from build123d import *

# Parameters (mm, degrees)
EXTRUDE_1_DEPTH     = 15
SKETCH_3_W          = 10.742953118
SKETCH_3_H          = 10
EXTRUDE_2_DEPTH     = 57.5
SKETCH_4_W          = 10.742953118
SKETCH_4_H          = 5
EXTRUDE_3_DEPTH     = 57.5
CUT_EXTRUDE_1_REACH = 133.077
SKETCH_5_R          = 1.65
CUT_EXTRUDE_2_REACH = 137.116
SKETCH_6_R          = 1.7
CUT_EXTRUDE_3_REACH = 135.143
SKETCH_7_R          = 1.5
CHAMFER_1_SIZE      = 5
CHAMFER_2_SIZE      = 2
CHAMFER_3_SIZE      = 5
CHAMFER_4_SIZE      = 1


with BuildPart() as part:
    # Sketch 1 → Extrude 1 (new body)
    with BuildSketch(Plane.XY):
        Polygon((0, 110), (0, 0), (-30, 0), (-30, 5), (-20, 5), (-10.742953118, 14.257046882), (-10.742953118, 110), align=None)
    extrude(amount=EXTRUDE_1_DEPTH)


with BuildPart() as body_2:
    # Mirror 9: mirrored copy
    add(part.part.mirror(Plane.XY.offset(-28.75)))


with BuildPart() as part_1:
    add(part.part)

    add(body_2.part)  # Extrude 2 merges body 2
    # Sketch 3 → Extrude 2 (add)
    with BuildSketch(Plane.XY.offset(-57.5)):
        with Locations((-5.371476559, 75)):
            Rectangle(SKETCH_3_W, SKETCH_3_H)
    extrude(amount=EXTRUDE_2_DEPTH)

    # Sketch 4 → Extrude 3 (add)
    with BuildSketch(Plane.XY.offset(-57.5)):
        with Locations((-5.371476559, 2.5)):
            Rectangle(SKETCH_4_W, SKETCH_4_H)
    extrude(amount=EXTRUDE_3_DEPTH)

    # Sketch 5 → Cut-Extrude 1 (cut, up to next)
    with BuildSketch(Plane(origin=(0, 5, 0), x_dir=(1, 0, 0), z_dir=(0, 1, 0)), mode=Mode.PRIVATE) as cut_extrude_1_sk1:
        with Locations(Location((-24.537178605, 65, 0), (0, 0, 270))):
            Circle(SKETCH_5_R)
    cut_extrude_1_tool1 = extrude(cut_extrude_1_sk1.sketch, amount=-CUT_EXTRUDE_1_REACH, mode=Mode.PRIVATE) & part_1.part
    # Sketch 5 → Cut-Extrude 1 (cut, up to next)
    with BuildSketch(Plane(origin=(0, 5, 0), x_dir=(1, 0, 0), z_dir=(0, 1, 0)), mode=Mode.PRIVATE) as cut_extrude_1_sk2:
        with Locations(Location((-24.537178605, -7.5, 0), (0, 0, 270))):
            Circle(SKETCH_5_R)
    cut_extrude_1_tool2 = extrude(cut_extrude_1_sk2.sketch, amount=-CUT_EXTRUDE_1_REACH, mode=Mode.PRIVATE) & part_1.part
    add(cut_extrude_1_tool1.solids().sort_by_distance((-24.537179, 5, -65))[0], mode=Mode.SUBTRACT)
    add(cut_extrude_1_tool2.solids().sort_by_distance((-24.537179, 5, 7.5))[0], mode=Mode.SUBTRACT)

    # Sketch 6 → Cut-Extrude 2 (cut, up to next)
    with BuildSketch(Plane.XZ, mode=Mode.PRIVATE) as cut_extrude_2_sk1:
        with Locations((-4.537178605, -7.5)):
            Circle(SKETCH_6_R)
    cut_extrude_2_tool1 = extrude(cut_extrude_2_sk1.sketch, amount=-CUT_EXTRUDE_2_REACH, mode=Mode.PRIVATE) & part_1.part
    # Sketch 6 → Cut-Extrude 2 (cut, up to next)
    with BuildSketch(Plane.XZ, mode=Mode.PRIVATE) as cut_extrude_2_sk2:
        with Locations((-4.537178605, -50)):
            Circle(SKETCH_6_R)
    cut_extrude_2_tool2 = extrude(cut_extrude_2_sk2.sketch, amount=-CUT_EXTRUDE_2_REACH, mode=Mode.PRIVATE) & part_1.part
    add(cut_extrude_2_tool1.solids().sort_by_distance((-4.537179, 0, -7.5))[0], mode=Mode.SUBTRACT)
    add(cut_extrude_2_tool2.solids().sort_by_distance((-4.537179, 0, -50))[0], mode=Mode.SUBTRACT)

    # Sketch 7 → Cut-Extrude 3 (cut, up to next)
    with BuildSketch(Plane.ZY.offset(10.742953118), mode=Mode.PRIVATE) as cut_extrude_3_sk1:
        with Locations((-66.25, 100.05)):
            Circle(SKETCH_7_R)
    cut_extrude_3_tool1 = extrude(cut_extrude_3_sk1.sketch, amount=-CUT_EXTRUDE_3_REACH, mode=Mode.PRIVATE) & part_1.part
    # Sketch 7 → Cut-Extrude 3 (cut, up to next)
    with BuildSketch(Plane.ZY.offset(10.742953118), mode=Mode.PRIVATE) as cut_extrude_3_sk2:
        with Locations((8.75, 100.05)):
            Circle(SKETCH_7_R)
    cut_extrude_3_tool2 = extrude(cut_extrude_3_sk2.sketch, amount=-CUT_EXTRUDE_3_REACH, mode=Mode.PRIVATE) & part_1.part
    # Sketch 7 → Cut-Extrude 3 (cut, up to next)
    with BuildSketch(Plane.ZY.offset(10.742953118), mode=Mode.PRIVATE) as cut_extrude_3_sk3:
        with Locations((-66.25, 78.05)):
            Circle(SKETCH_7_R)
    cut_extrude_3_tool3 = extrude(cut_extrude_3_sk3.sketch, amount=-CUT_EXTRUDE_3_REACH, mode=Mode.PRIVATE) & part_1.part
    # Sketch 7 → Cut-Extrude 3 (cut, up to next)
    with BuildSketch(Plane.ZY.offset(10.742953118), mode=Mode.PRIVATE) as cut_extrude_3_sk4:
        with Locations(Location((8.75, 78.05, 0), (0, 0, 270))):
            Circle(SKETCH_7_R)
    cut_extrude_3_tool4 = extrude(cut_extrude_3_sk4.sketch, amount=-CUT_EXTRUDE_3_REACH, mode=Mode.PRIVATE) & part_1.part
    add(cut_extrude_3_tool1.solids().sort_by_distance((-10.742953, 100.05, -66.25))[0], mode=Mode.SUBTRACT)
    add(cut_extrude_3_tool2.solids().sort_by_distance((-10.742953, 100.05, 8.75))[0], mode=Mode.SUBTRACT)
    add(cut_extrude_3_tool3.solids().sort_by_distance((-10.742953, 78.05, -66.25))[0], mode=Mode.SUBTRACT)
    add(cut_extrude_3_tool4.solids().sort_by_distance((-10.742953, 78.05, 8.75))[0], mode=Mode.SUBTRACT)

    # Chamfer 1
    chamfer_1_edges = [part_1.edges().sort_by_distance(p)[0] for p in [
        (-5.371476559, 80, 0),
        (-5.371476559, 80, -57.5),
        (-5.371476559, 70, 0),
        (-5.371476559, 70, -57.5),
        (-5.371476559, 5, 0),
        (-5.371476559, 5, -57.5),
    ]]
    chamfer(chamfer_1_edges, length=CHAMFER_1_SIZE)

    # Chamfer 2
    chamfer_2_edges = [part_1.edges().sort_by_distance(p)[0] for p in [
        (-5.371476559, 110, 0),
        (-30, 2.5, 15),
        (-5.371476559, 110, -57.5),
        (-30, 2.5, -57.5),
        (-5.371476559, 110, -72.5),
        (-30, 2.5, -72.5),
        (-5.371476559, 110, 15),
        (-30, 2.5, 0),
    ]]
    chamfer(chamfer_2_edges, length=CHAMFER_2_SIZE)

    # Chamfer 3
    # the kernel refuses this chamfer: 5 mm, written as the material it adds along each edge
    with BuildSketch(Plane(origin=(-10.742953118, 22.85841494, 0), x_dir=(-0.9996219169112968, 0, 0.027495876610586372), z_dir=(0, -1, 0))) as chamfer_3_piece_1_section:
        Polygon((CHAMFER_3_SIZE * 0.999621916911, CHAMFER_3_SIZE * 0.0274958766106), (-CHAMFER_3_SIZE * 0.0274958766106, CHAMFER_3_SIZE * 0.999621916911), (0, 0), align=None)
    chamfer_3_piece_1 = extrude(amount=22.85841494, mode=Mode.PRIVATE)
    chamfer_3_piece_1 = split(chamfer_3_piece_1, bisect_by=Plane(origin=(-12.636913345, 5, -1.178868923), z_dir=(0, 1, 0)), keep=Keep.TOP, mode=Mode.PRIVATE)
    chamfer_3_piece_1 = split(chamfer_3_piece_1, bisect_by=Plane(origin=(-12.636913345, 7.862667434, -2.137332566), z_dir=(0, -0.7071067811865476, 0.7071067811865476)), keep=Keep.TOP, mode=Mode.PRIVATE)
    chamfer_3_piece_1 = split(chamfer_3_piece_1, bisect_by=Plane(origin=(-15.366354777, 9.633645223, -1.178868923), z_dir=(0.7071067811865488, -0.7071067811865464, 0)), keep=Keep.TOP, mode=Mode.PRIVATE)
    add(chamfer_3_piece_1)
    with BuildSketch(Plane(origin=(-10.742953118, 22.85841494, 0), x_dir=(-0.9996219169112968, 0, 0.027495876610586372), z_dir=(0, -1, 0))) as chamfer_3_piece_2_section:
        Polygon((CHAMFER_3_SIZE * 0.999621916911, CHAMFER_3_SIZE * 0.0274958766106), (-CHAMFER_3_SIZE * 0.0274958766106, CHAMFER_3_SIZE * 0.999621916911), (0, 0), align=None)
    chamfer_3_piece_2 = extrude(amount=22.85841494, mode=Mode.PRIVATE)
    chamfer_3_piece_2 = split(chamfer_3_piece_2, bisect_by=Plane(origin=(-12.391958981, 5, -1.648896507), z_dir=(0, -1, 0)), keep=Keep.TOP, mode=Mode.PRIVATE)
    chamfer_3_piece_2 = split(chamfer_3_piece_2, bisect_by=Plane(origin=(-12.391958981, 5.425526159, -4.574473841), z_dir=(0, -0.7071067811865476, 0.7071067811865476)), keep=Keep.TOP, mode=Mode.PRIVATE)
    add(chamfer_3_piece_2)
    with BuildSketch(Plane(origin=(-10.742953118, 0, -57.5), x_dir=(-0.9996219169112968, 0, -0.027495876610586317), z_dir=(0, 1, 0))) as chamfer_3_piece_3_section:
        Polygon((CHAMFER_3_SIZE * 0.999621916911, CHAMFER_3_SIZE * 0.0274958766106), (-CHAMFER_3_SIZE * 0.0274958766106, CHAMFER_3_SIZE * 0.999621916911), (0, 0), align=None)
    chamfer_3_piece_3 = extrude(amount=22.85841494, mode=Mode.PRIVATE)
    chamfer_3_piece_3 = split(chamfer_3_piece_3, bisect_by=Plane(origin=(-12.391958981, 5.425526159, -52.925526159), z_dir=(0, -0.7071067811865476, -0.7071067811865476)), keep=Keep.TOP, mode=Mode.PRIVATE)
    chamfer_3_piece_3 = split(chamfer_3_piece_3, bisect_by=Plane(origin=(-12.391958981, 5, -55.851103493), z_dir=(0, -1, 0)), keep=Keep.TOP, mode=Mode.PRIVATE)
    add(chamfer_3_piece_3)
    with BuildSketch(Plane(origin=(-10.742953118, 0, -57.5), x_dir=(-0.9996219169112968, 0, -0.027495876610586317), z_dir=(0, 1, 0))) as chamfer_3_piece_4_section:
        Polygon((CHAMFER_3_SIZE * 0.999621916911, CHAMFER_3_SIZE * 0.0274958766106), (-CHAMFER_3_SIZE * 0.0274958766106, CHAMFER_3_SIZE * 0.999621916911), (0, 0), align=None)
    chamfer_3_piece_4 = extrude(amount=22.85841494, mode=Mode.PRIVATE)
    chamfer_3_piece_4 = split(chamfer_3_piece_4, bisect_by=Plane(origin=(-12.636913345, 7.862667434, -55.362667434), z_dir=(0, -0.7071067811865476, -0.7071067811865476)), keep=Keep.TOP, mode=Mode.PRIVATE)
    chamfer_3_piece_4 = split(chamfer_3_piece_4, bisect_by=Plane(origin=(-15.366354777, 9.633645223, -56.321131077), z_dir=(0.7071067811865488, -0.7071067811865464, 0)), keep=Keep.TOP, mode=Mode.PRIVATE)
    chamfer_3_piece_4 = split(chamfer_3_piece_4, bisect_by=Plane(origin=(-12.636913345, 5, -56.321131077), z_dir=(0, 1, 0)), keep=Keep.TOP, mode=Mode.PRIVATE)
    add(chamfer_3_piece_4)

    # Chamfer 4
    chamfer_4_edges = [part_1.edges().sort_by_distance(p)[0] for p in [
        (-10.742953118, 39.628523441, 0),
        (-10.742953118, 39.628523441, -57.5),
        (-10.742953118, 70, -28.75),
        (-10.742953118, 80, -28.75),
        (-10.742953118, 67.5, -55),
        (-10.742953118, 67.5, -2.5),
        (-10.742953118, 82.5, -2.5),
        (-10.742953118, 82.5, -55),
        (-15.371476559, 9.628523441, 15),
        (-10.742953118, 61.128523441, 15),
        (-24, 5, 15),
        (-30, 5, 7.5),
        (-29, 5, 1),
        (-29, 5, 14),
        (-30, 5, -65),
        (-29, 5, -71.5),
        (-29, 5, -58.5),
        (-10.742953118, 61.128523441, -72.5),
        (-10.742953118, 96.5, 0),
        (-10.742953118, 96.5, -57.5),
        (-10.742953118, 110, -65),
        (-10.742953118, 110, 7.5),
        (-10.742953118, 109, -71.5),
        (-10.742953118, 109, -58.5),
        (-10.742953118, 109, 1),
        (-10.742953118, 109, 14),
        (-17.871476559, 7.128523441, 0),
        (-17.871476559, 7.128523441, -57.5),
        (-12.871476559, 12.128523441, -57.5),
        (-24, 5, -57.5),
        (-15.371476559, 9.628523441, -72.5),
        (-24, 5, -72.5),
        (-24, 5, 0),
        (-12.871476559, 12.128523441, 0),
    ]]
    chamfer(chamfer_4_edges, length=CHAMFER_4_SIZE)


solid = part_1.part
For this review, take the finished solid that the model builds, in its own axes (mm). A direction names the side the tool comes from. Coordinates: 2 decimals unless noted, no trailing zeros. Order: outer loops, then holes, each group sorted by start corner. A loop starts at its lowest first (then second) coordinate and runs counter-clockwise, first axis right, second up. Notation, with made-up numbers: (14, 62.5) - (25, 62.5) arc R13 ccw to (25, 67.5) - close; hole circle Ø2 at (-11.75, -11.5). An arc over 180 degrees is marked (long way). Use one line per item in the form item = value.
Q1. Consider section C-C (x = -8). Give the boundary of the cut face in (y, z).
Checked values:
outline = (0, -72.5) - (108, -72.5) - (110, -70.5) - (110, -59.5) - (108, -57.5) - (85, -57.5) - (80, -52.5) - (80, -5) - (85, 0) - (108, 0) - (110, 2) - (110, 13) - (108, 15) - (0, 15) - close; hole (5, -52.5) - (10, -57.5) - (65, -57.5) - (70, -52.5) - (70, -5) - (65, 0) - (10, 0) - (5, -5) - close; hole circle Ø3 at (78.05, -66.25); hole circle Ø3 at (78.05, 8.75); hole circle Ø3 at (100.05, -66.25); hole circle Ø3 at (100.05, 8.75)
Q2. For faces 1 (the flat face through (-12.04, 12.24, -57.99)), 2 (the flat face through (-4.9, 82.5, -55)), 3 (the flat face through (-10.25, 82.1, -55.32)), 4 (the flat face through (-5, 38, 0)), list the 3-axis set-ups (+Z, -Z, +X, -X, +Y, -Y) from which the entire face can be reached by the end or side of a thin tool; tool diameter is ignored.
Checked values:
face_1 = -X
face_2 = +X, -X, +Y
face_3 = -X, +Y
face_4 = +X, -X
Q3. Consider section D-D (z = -18). Give the boundary of the cut face in (x, y).
Checked values:
outline = (-10.74, 0) - (0, 0) - (0, 5) - (-10.74, 5) - close; (-10.74, 71) - (-9.74, 70) - (0, 70) - (0, 80) - (-9.74, 80) - (-10.74, 79) - close
Q4. Consider section A-A (y = 23.5). Give the boundary of the cut face in (x, z).
Checked values:
outline = (-10.74, -71.5) - (-9.74, -72.5) - (0, -72.5) - (0, -57.5) - (-9.74, -57.5) - (-10.74, -58.5) - close; (-10.74, 1) - (-9.74, 0) - (0, 0) - (0, 15) - (-9.74, 15) - (-10.74, 14) - close
Q5. For P1, Ø4, axis at y = 78.05, z = 8.75, coming from the -X side; P2, Ø12, axis at x = -7.5, z = -39.5, coming from the +Y side; P3, Ø3, axis at x = -24.5, z = 3.5, coming from the +Y side, all flat-tipped, find the tip position at first contact; note any pin that passes through.
Checked values:
P1 = -10.74
P2 = 80
P3 = 5
Q6. For probe 1 along Z at (x, y) = (-2.75, 100.05); probe 2 along Z at (x, y) = (-5.5, 78.05); probe 3 along Y at (x, z) = (-8, 8.5), list the stretches that pass through material, from the lowest coordinate up. Write a range as from..to.
Checked values:
probe_1 = -72.5..-67.75, -64.75..-57.5, 0..7.25, 10.25..15
probe_2 = -72.5..-67.75, -64.75..7.25, 10.25..15
probe_3 = 0..76.57, 79.53..98.57, 101.53..110
Q7. Consider section B-B (y = 100.05). Give the boundary of the cut face in (x, z).
Checked values:
outline = (-10.74, -71.5) - (-9.74, -72.5) - (0, -72.5) - (0, -67.75) - (-10.74, -67.75) - close; (-10.74, -64.75) - (0, -64.75) - (0, -57.5) - (-9.74, -57.5) - (-10.74, -58.5) - close; (-10.74, 1) - (-9.74, 0) - (0, 0) - (0, 7.25) - (-10.74, 7.25) - close; (-10.74, 10.25) - (0, 10.25) - (0, 15) - (-9.74, 15) - (-10.74, 14) - close
Q8. Draft analysis for pull direction Z (two halves, no side actions). For faces 5 (the flat face through (-10.25, 108.655, -71.127)), 6 (the flat face through (-10.743, 72, -29)), 7 (the cylindrical face through (-5.4, 98.7, 9.4)), state which applies: +Z half, -Z half, draft (parallel to the pull), parting line (faces both ways), or undercut.
Checked values:
face_5 = -Z half
face_6 = draft
face_7 = undercut
